```python
from build123d import *

# Parameters (mm, degrees)
SKETCH2_W           = 128
SKETCH2_H           = 150
SKETCH2_W_2         = 24.5
SKETCH2_H_2         = 10
BOSS_EXTRUDE1_DEPTH = 20


with BuildPart() as part:
    # Sketch2 → Boss-Extrude1 (new body)
    with BuildSketch(Plane.XY):
        Rectangle(SKETCH2_W, SKETCH2_H)
        with Locations((-31.75, -50)):
            Rectangle(SKETCH2_W_2, SKETCH2_H_2, mode=Mode.SUBTRACT)
        with Locations((31.75, -50)):
            Rectangle(SKETCH2_W_2, SKETCH2_H_2, mode=Mode.SUBTRACT)
    extrude(amount=BOSS_EXTRUDE1_DEPTH)


solid = part.part
```
Can you work these out from the model? Positions are in its coordinate system, mm. A direction names the side the tool comes from. Give positions to 0.01 mm unless a question says otherwise; leave off trailing zeros. Write each loop counter-clockwise with the first axis right and the second up, starting at its lowest first coordinate (ties: lowest second). Pieces come first, ordered by that corner, then holes. Notation, with made-up numbers: (59, 13.25) -> (67, 13.25) arc R20 cw to (67, 25.25) -> close; hole circle Ø3 at (40, 26). An arc over 180 degrees is marked (long way). One line per item, written item: value.
Q1. Which directions (+Z, -Z, +X, -X, +Y, -Y) give clear straight access to the entire face, cutting with the end or side of a thin tool? Please do faces 5 (the face through (-19.5, -50, 10)), 6 (the face through (-1, 1, 20)).
Results found:
face 5: +Z, -Z
face 6: +Z, +X, -X, +Y, -Y
Q2. Imagine slicing it at A-A on x = -33.5. Please give me the cut outline in (y, z).
Results found:
outline: (-75, 0) -> (-55, 0) -> (-55, 20) -> (-75, 20) -> close; (-45, 0) -> (75, 0) -> (75, 20) -> (-45, 20) -> close
Q3. Imagine slicing it at B-B on z = 16. Please give me the cut outline in (x, y).
Results found:
outline: (-64, -75) -> (64, -75) -> (64, 75) -> (-64, 75) -> close; hole (-44, -55) -> (-19.5, -55) -> (-19.5, -45) -> (-44, -45) -> close; hole (19.5, -55) -> (44, -55) -> (44, -45) -> (19.5, -45) -> close
Q4. Please list where these lines run through material, in increasing order: line 1 (X direction, y = -50, z = 18.25); line 2 (Y direction, x = -37, z = 4). Write a range as [from, to].
Results found:
line 1: x = [-64, -44], [-19.5, 19.5], [44, 64]
line 2: y = [-75, -55], [-45, 75]
Q5. We'd pull the mould along Y, two halves only. Please class faces 1 (the face through (-1, -75, 10)), 2 (the face through (-1, 75, 10)), 3 (the face through (32, -55, 10)), 4 (the face through (64, -1, 10)): +Y half, -Y half, draft (parallel to the pull), parting line (faces both ways), or undercut.
Results found:
face 1: -Y half
face 2: +Y half
face 3: undercut
face 4: draft
